from build123d import *

# Parameters (mm, degrees)
SKETCH1_R           = 5.07
SKETCH1_R_2         = 4
BOSS_EXTRUDE1_DEPTH = 10.3
SKETCH1_3_R         = 11
SKETCH1_3_R_2       = 5.07
SKETCH1_3_R_3       = 4
BOSS_EXTRUDE2_DEPTH = 3.7
SKETCH2_R           = 5.07
SKETCH2_R_2         = 4
BOSS_EXTRUDE3_DEPTH = 1.5
CHAMFER1_SIZE       = 0.508
SKETCH3_R           = 1.7
CUT_EXTRUDE1_DEPTH  = 4.294


with BuildPart() as part:
    # Sketch1 → Boss-Extrude1 (new body)
    with BuildSketch(Plane.XY):
        with Locations(Location((0, 0, 0), (0, 0, 180))):
            Circle(SKETCH1_R)
        with Locations(Location((0, 0, 0), (0, 0, 180))):
            Circle(SKETCH1_R_2, mode=Mode.SUBTRACT)
    extrude(amount=BOSS_EXTRUDE1_DEPTH)

    # Sketch1<3> → Boss-Extrude2 (add)
    with BuildSketch(Plane.XY):
        Circle(SKETCH1_3_R)
        with Locations(Location((0, 0, 0), (0, 0, 180))):
            Circle(SKETCH1_3_R_2, mode=Mode.SUBTRACT)
        with Locations(Location((0, 0, 0), (0, 0, 180))):
            Circle(SKETCH1_3_R_2)
        with Locations(Location((0, 0, 0), (0, 0, 180))):
            Circle(SKETCH1_3_R_3, mode=Mode.SUBTRACT)
    extrude(amount=-BOSS_EXTRUDE2_DEPTH)

    # Sketch2 → Boss-Extrude3 (add)
    with BuildSketch(Plane(origin=(0, 0, -3.7), x_dir=(-1, 0, 0), z_dir=(0, 0, -1))):
        Circle(SKETCH2_R)
        Circle(SKETCH2_R_2, mode=Mode.SUBTRACT)
    extrude(amount=BOSS_EXTRUDE3_DEPTH)

    # Chamfer1
    chamfer1_edges = [part.edges().sort_by_distance(p)[0] for p in [
        (4, 0, -5.2),
        (4, 0, 10.3),
    ]]
    chamfer(chamfer1_edges, length=CHAMFER1_SIZE)

    # Sketch3 → Cut-Extrude1 (cut)
    with BuildSketch(Plane(origin=(0, 0, -3.7), x_dir=(-1, 0, 0), z_dir=(0, 0, -1))):
        with Locations((-8.035, 0)):
            Circle(SKETCH3_R)
        with Locations((0, 8.035)):
            Circle(SKETCH3_R)
        with Locations((8.035, 0)):
            Circle(SKETCH3_R)
        with Locations((0, -8.035)):
            Circle(SKETCH3_R)
    extrude(amount=-CUT_EXTRUDE1_DEPTH, mode=Mode.SUBTRACT)


solid = part.part
Read the model definition and answer for the solid it produces. Units are mm, in the model's axes. A direction names the side the tool comes from. Coordinates: 2 decimals unless noted, no trailing zeros. Loops run counter-clockwise (first coordinate to the right, second up) from the corner with the lowest first, then second, coordinate; pieces in that order, holes last.
Q1. The mould has two halves that part along Y. Classify faces 1 (the face through (2, -5, 0)), 2 (the face through (-6.337, 0.075, -1.876)), 3 (the face through (-4.836, 1.523, -4.44)): +Y half, -Y half, draft (parallel to the pull), parting line (faces both ways), or undercut.
Q2. The part is cut by section D-D on x = 7.75. Write down the section's boundary in (y, z).
Q3. The part is cut by section A-A on x = 0. Write down the section's boundary in (y, z) (3 decimals).
Q4. Consider probe 1 along Y at (x, z) = (0, -0.9) (3 decimals); probe 2 along Z at (x, y) = (8.5, -5.25); probe 3 along X at (y, z) = (-1.75, -2.75). Determine where each line is inside the solid, lowest interval first.
Q5. The part is cut by section C-C on z = -3.25. Write down the section's boundary in (x, y) (3 decimals), and give its area (3 significant figures).
Q6. Which of the six approach directions +Z, -Z, +X, -X, +Y, -Y give full straight-line access (tool end or side, diameter ignored) to faces 4 (the face through (-4.836, -1.523, 5.078)), 5 (the face through (2, -5, -3.7)), 6 (the face through (0.22, 9.72, -1.88))?
Q7. Each of these flat-tipped pins is pushed along its axis until it touches: pin 1 Ø4 at (x, y) = (-2.5, 7.5) entering from -Z; pin 2 Ø5.5 at (x, y) = (-8.035, 0) entering from +Z; pin 3 Ø3 at (x, z) = (4, 4) entering from +Y. Where does it stop, or does it pass through?
Results below:
1. face 1: draft
1. face 2: undercut
1. face 3: parting line
2. outline: (-7.81, -3.7) - (-1.68, -3.7) - (-1.68, 0) - (-7.81, 0) - close; (1.68, -3.7) - (7.81, -3.7) - (7.81, 0) - (1.68, 0) - close
3. outline: (-11, -3.7) - (-9.735, -3.7) - (-9.735, 0) - (-11, 0) - close; (-6.335, -3.7) - (-5.07, -3.7) - (-5.07, -5.2) - (-4.508, -5.2) - (-4, -4.692) - (-4, 9.792) - (-4.508, 10.3) - (-5.07, 10.3) - (-5.07, 0) - (-6.335, 0) - close; (4, -4.692) - (4.508, -5.2) - (5.07, -5.2) - (5.07, -3.7) - (6.335, -3.7) - (6.335, 0) - (5.07, 0) - (5.07, 10.3) - (4.508, 10.3) - (4, 9.792) - close; (9.735, -3.7) - (11, -3.7) - (11, 0) - (9.735, 0) - close
4. probe 1: y = -11 to -9.735, -6.335 to -4, 4 to 6.335, 9.735 to 11
4. probe 2: z = -3.7 to 0
4. probe 3: x = -10.86 to -3.6, 3.6 to 10.86
5. outline: circle Ø22 at (0, 0); hole circle Ø3.4 at (-8.035, 0); hole circle Ø8 at (0, 0); hole circle Ø3.4 at (0, -8.035); hole circle Ø3.4 at (0, 8.035); hole circle Ø3.4 at (8.035, 0)
5. area: 294 mm2
6. face 4: +Z
6. face 5: -Z
6. face 6: +Z, -Z
7. pin 1: stops at z = -3.7
7. pin 2: stops at z = 0
7. pin 3: stops at y = 4.41
